Can you work these out from the model? Positions are in its coordinate system, mm. Face numbers are marked on the shaded views. Round coordinates to 2 decimals unless told otherwise and drop trailing zeros. Write each loop counter-clockwise with the first axis right and the second up, starting at its lowest first coordinate (ties: lowest second). Pieces come first, ordered by that corner, then holes. Notation, with made-up numbers: M 83.5,51 L 87.5,51 A15 cw 87.5,64 Z; hole C 48,-39.75 d7. An arc over 180 degrees is marked long. Answer as a JSON object with one key per item and string values. Group by question number.
1) Please list where these lines run through material, in increasing order: L1, parallel to X at y = 12, z = -0.65; L2, parallel to Y at x = -6, z = 0.65; L3, parallel to X at y = 17, z = 1.9. Write a range as [from, to].
2) If we mould it in two halves opening along X, with no side actions, what happens to the marked faces 1 and 2? For each: +X half, -X half, draft (parallel to the pull), parting line (faces both ways), or undercut.
3) I'm going to push flat-ended pins straight in: pin 1 Ø1.1 at (x, z) = (-22, 0) entering from +Y; pin 2 Ø2 at (x, z) = (7.5, -1) entering from +Y (3 decimals); pin 3 Ø3.5 at (x, y) = (35.5, -3.5) entering from +Z. Where does each tip first touch, or does it pass through?
4) Suppose I cut it at B-B, the plane x = -24. Write out the boundary of the cut face in (y, z).
5) Suppose I cut it at A-A, the plane y = 0. Write out the boundary of the cut face in (x, z), and give its area (3 significant figures).
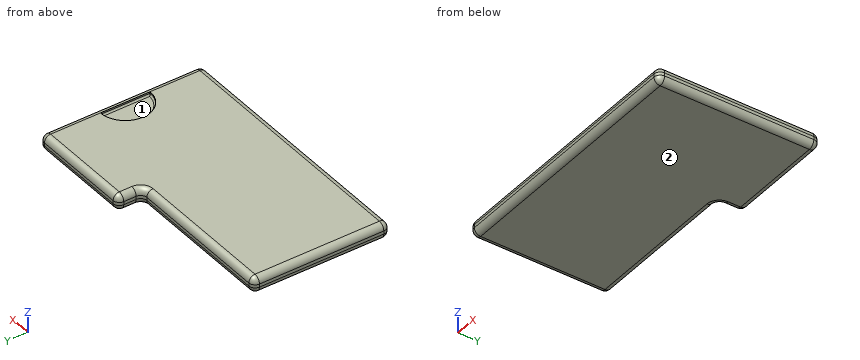
from build123d import *

# Parameters (mm, degrees)
SALIENTE_EXTRUIR1_DEPTH = 2.5
REDONDEO1_R             = 2
CORTAR_EXTRUIR1_DEPTH   = 1
REDONDEO2_R             = 0.5


with BuildPart() as part:
    # Croquis1 → Saliente-Extruir1 (new body, symmetric)
    with BuildSketch(Plane.XY):
        Polygon((7.5, 26), (42.5, 26), (42.5, -26), (-42.5, -26), (-42.5, 18), (-7.5, 18), (7.5, 18), align=None)
    extrude(amount=SALIENTE_EXTRUIR1_DEPTH, both=True)

    # Redondeo1
    redondeo1_edges = [part.edges().sort_by_distance(p)[0] for p in [
        (42.5, 0, -2.5),
        (42.5, -26, 0),
        (-42.5, -26, 0),
        (-42.5, 18, 0),
        (7.5, 22, 2.5),
        (7.5, 18, 0),
        (7.5, 26, 0),
        (42.5, 26, 0),
        (-17.5, 18, 2.5),
        (-42.5, -4, 2.5),
        (0, -26, 2.5),
        (42.5, 0, 2.5),
        (0, -26, -2.5),
        (-42.5, -4, -2.5),
        (-17.5, 18, -2.5),
        (25, 26, 2.5),
        (7.5, 22, -2.5),
        (25, 26, -2.5),
    ]]
    fillet(redondeo1_edges, radius=REDONDEO1_R)

    # Croquis2 → Cortar-Extruir1 (cut)
    with BuildSketch(Plane.XY.offset(2.5)):
        with BuildLine():
            Line((40.5, 8), (40.5, -8))
            ThreePointArc((40.5, -8), (32.5, 0), (40.5, 8))
        make_face()
    extrude(amount=-CORTAR_EXTRUIR1_DEPTH, mode=Mode.SUBTRACT)

    # Redondeo2
    redondeo2_edges = [part.edges().sort_by_distance(p)[0] for p in [
        (32.5, 0, 1.5),
        (40.5, 0, 1.5),
    ]]
    fillet(redondeo2_edges, radius=REDONDEO2_R)


solid = part.part
Results:
{
 "1": {"L1": "[-42.49, 42.49]", "L2": "[-25.99, 17.99]", "L3": "[-41.52, 41.93]"},
 "2": {"face 1": "undercut", "face 2": "draft"},
 "3": {"pin 1": "y = 18", "pin 2": "y = 25.695", "pin 3": "z = 1.65"},
 "4": {"outline": "M -26,-0.5 A2 ccw -24,-2.5 L 16,-2.5 A2 ccw 18,-0.5 L 18,0.5 A2 ccw 16,2.5 L -24,2.5 A2 ccw -26,0.5 Z"},
 "5": {"outline": "M -42.5,-0.5 A2 ccw -40.5,-2.5 L 40.5,-2.5 A2 ccw 42.5,-0.5 L 42.5,0.5 A2 ccw 40.5,2.5 L 40.5,2 A0.5 cw 40,1.5 L 33,1.5 A0.5 cw 32.5,2 L 32.5,2.5 L -40.5,2.5 A2 ccw -42.5,0.5 Z", "area": "414 mm^2"}
}
